Geometry: final body of the model. Coordinates: model frame, mm. A direction names the side the tool comes from. Coordinates: 2 decimals unless noted, no trailing zeros. Order: outer loops, then holes, each group sorted by start corner. A loop starts at its lowest first (then second) coordinate and runs counter-clockwise, first axis right, second up. Notation, with made-up numbers: M 13.25,53 L 69.25,53 A21 cw 69.25,88 Z; hole C 61,50.5 d5. An arc over 180 degrees is marked long. Use CSV: the item, a comma, the result in double quotes. Start each with the question number.
Q1. Section query B-B, the plane x = 9.5. Output: boundary loops of the cut face in (y, z), and give its area (3 significant figures).
Q2. Section query C-C, the plane y = 15.5. Output: boundary loops of the cut face in (x, z).
Q3. Access query for faces 1 (the face through (0, 8, 24)), 2 (the face through (12, 2, 11)). Directions: +Z, -Z, +X, -X, +Y, -Y. A direction counts if a zero-diameter tool reaches every point of the face in a straight line with its end or side. Return the directions, or none.
Q4. Mould query, pull axis Z, two halves, no side actions, for faces 3 (the face through (11.52, 1.01, 12.4)), 4 (the face through (10, 12, 25.3)), 5 (the face through (20, 8, 24)). Classes: +Z half, -Z half, draft (parallel to the pull), parting line (faces both ways), or undercut.
Q5. Ray query, probe 1 along X at (y, z) = (0.7, 11.25); probe 2 along Y at (x, z) = (10, 24.65); probe 3 along Y at (x, z) = (19, 19.5). Return the intervals inside material, ascending.
Q6. Section query A-A, the plane z = 11.25. Output: boundary loops of the cut face in (x, y).
Q7. First-contact query: P1, Ø2, axis at x = 4, y = 11, coming from the -Z side; P2, Ø1.5, axis at x = 7.5, z = 17, coming from the +Y side. Flat tips, straight axial feed; report the tip coordinate or a pass-through.
Q8. Section query D-D, the plane x = 2.25. Output: boundary loops of the cut face in (y, z).
Autodesk Inventor part; units mm, degrees
ref_plane "YZ Plane" through (0, 0, 0) normal (1, 0, 0) x (0, 1, 0)
ref_plane "XZ Plane" through (0, 0, 0) normal (0, 1, 0) x (-1, 0, 0)
ref_plane "XY Plane" through (0, 0, 0) normal (0, 0, 1) x (1, 0, 0)
sketch "Esboço1" plane through (0, 0, 0) normal (0, 0, 1) x (1, 0, 0)
  line L0 (0, 0) -> (20, 0)
  line L1 (20, 0) -> (20, 2)
  line L2 (20, 2) -> (0, 2)
  line L3 (0, 2) -> (0, 0)
  dimension "d0" = 20
  dimension "d1" = 2
extrude "Extrusão1" add sketch "Esboço1" along normal blind 25.3
sketch "Esboço2" plane through (0, 2, 0) normal (0, 1, 0) x (1, 0, 0)
  line L0 (0, -25.3) -> (20, -25.3)
  line L1 (0, 0) -> (0, -25.3)
  line L2 (20, -25.3) -> (0, -25.3)
  line L3 (0, -25.3) -> (0, -23.3)
  line L4 (0, -23.3) -> (20, -23.3)
  line L5 (20, -23.3) -> (20, -25.3)
  dimension "d4" = 2
extrude "Extrusão2" add sketch "Esboço2" along normal blind 28
sketch "Esboço3" plane through (0, 2, 0) normal (0, 1, 0) x (1, 0, 0)
  circle A0 centre (8.75, -11.25) radius 3
  line L0 (20, 0) -> (0, 0)
  line L1 (0, 0) -> (0, -23.3)
  dimension "d7" = 6
  dimension "d8" = 11.25
  dimension "d9" = 8.75
extrude "Extrusão3" cut sketch "Esboço3" against normal blind 28
sketch "Esboço4" plane through (20, 2, 23.3) normal (0, 0, -1) x (-1, 0, 0)
  circle A0 centre (10, 14.913) radius 3
  line L0 (20, 0) -> (20, 28)
  line L1 (0, 28) -> (20, 28)
  line L2 (0, 0) -> (20, 0)
  point P0 (20, -2)
  dimension "d12" = 6
  dimension "d13" = 10
  dimension "d17" = 14.913
extrude "Extrusão4" cut sketch "Esboço4" against normal blind 28
properties part number "Fixador acelerometro dianteiro"
Responses:
1,outline,"M 0,0 L 2,0 L 2,8.35 L 0,8.35 Z; M 0,14.15 L 2,14.15 L 2,23.3 L 13.95,23.3 L 13.95,25.3 L 0,25.3 Z; M 19.87,23.3 L 30,23.3 L 30,25.3 L 19.87,25.3 Z"
1,area,"83.1 mm²"
2,outline,"M 0,23.3 L 7.35,23.3 L 7.35,25.3 L 0,25.3 Z; M 12.65,23.3 L 20,23.3 L 20,25.3 L 12.65,25.3 Z"
3,face 1,"+Z, -Z, -X, +Y, -Y"
3,face 2,"-Z, +X, -X, +Y"
4,face 3,"undercut"
4,face 4,"+Z half"
4,face 5,"draft"
5,probe 1,"x = 0 to 5.75, 11.75 to 20"
5,probe 2,"y = 0 to 13.91, 19.91 to 30"
5,probe 3,"y = 0 to 2"
6,outline,"M 0,0 L 5.75,0 L 5.75,2 L 0,2 Z; M 11.75,0 L 20,0 L 20,2 L 11.75,2 Z"
7,P1,"stops at z = 23.3"
7,P2,"stops at y = 2"
8,outline,"M 0,0 L 2,0 L 2,23.3 L 30,23.3 L 30,25.3 L 0,25.3 Z"
